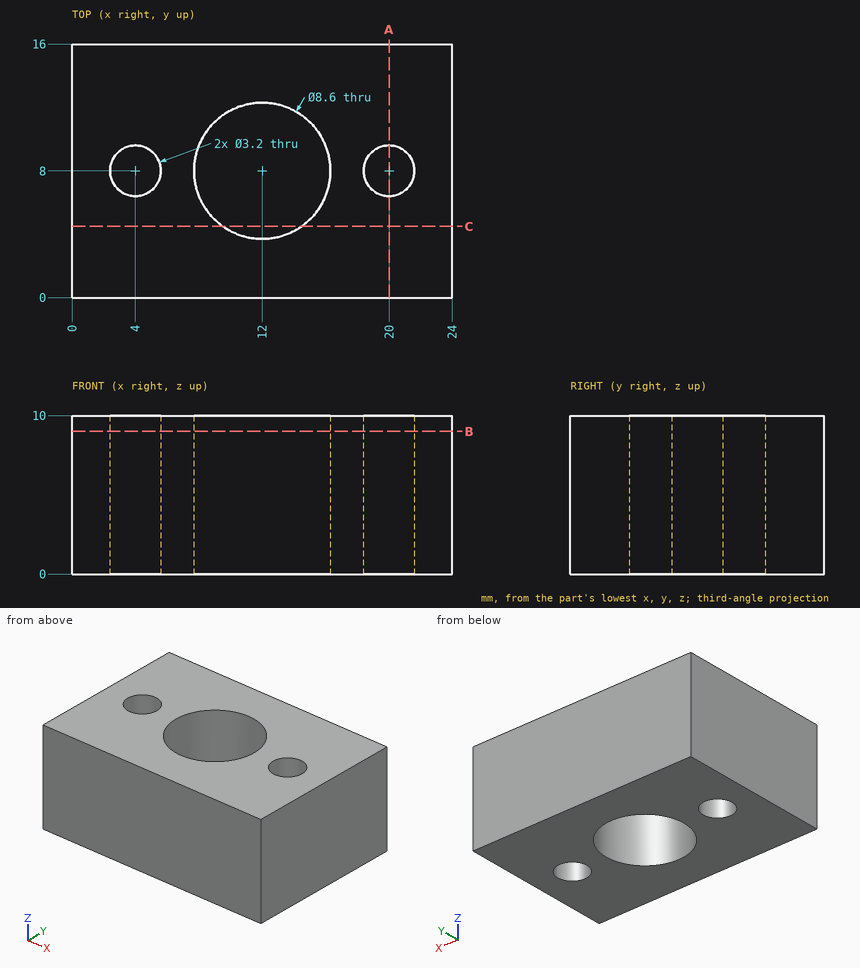
The drawing under review shows one solid part. Ordinate dimensions are in mm from its lowest x, y, z. Give positions to 0.01 mm unless a question says otherwise; leave off trailing zeros. Loops run counter-clockwise (first coordinate to the right, second up) from the corner with the lowest first, then second, coordinate; pieces in that order, holes last. Notation, with made-up numbers: M -34,14.25 L 6,14.25 A24 ccw 6,47.25 Z; hole C 60.5,52 d5. An arc over 180 degrees is marked long. Return JSON: item names as keys, results as strings. Group by question number.
Item 1: Insertion check: pin 1 Ø3 at (x, y) = (4, 8) entering from +Z. The pin has a flat end and moves straight along its axis. Give the tip position at first contact, or say it passes through.
Item 2: We need section B-B (z = 9). Give the boundary of the cut face in (x, y), and give its area (3 significant figures).
Item 3: We need section C-C (y = 4.5). Give the boundary of the cut face in (x, z), and give its area (3 significant figures).
Item 4: For probe 1 along X at (y, z) = (8, 6); probe 2 along Y at (x, z) = (12, 8); probe 3 along Y at (x, z) = (4, 6.25), list the stretches that pass through material, from the lowest coordinate up.
Item 5: We need section A-A (x = 20). Give the boundary of the cut face in (y, z), and give its area (3 significant figures).
Output:
{
 "1": {"pin 1": "passes through"},
 "2": {"outline": "M 0,0 L 24,0 L 24,16 L 0,16 Z; hole C 4,8 d3.2; hole C 12,8 d8.6; hole C 20,8 d3.2", "area": "310 mm^2"},
 "3": {"outline": "M 0,0 L 9.5,0 L 9.5,10 L 0,10 Z; M 14.5,0 L 24,0 L 24,10 L 14.5,10 Z", "area": "190 mm^2"},
 "4": {"probe 1": "x = 0 to 2.4, 5.6 to 7.7, 16.3 to 18.4, 21.6 to 24", "probe 2": "y = 0 to 3.7, 12.3 to 16", "probe 3": "y = 0 to 6.4, 9.6 to 16"},
 "5": {"outline": "M 0,0 L 6.4,0 L 6.4,10 L 0,10 Z; M 9.6,0 L 16,0 L 16,10 L 9.6,10 Z", "area": "128 mm^2"}
}
